Part model, mm, in its own coordinate system. A direction names the side the tool comes from. Round coordinates to 2 decimals unless told otherwise and drop trailing zeros. Write each loop counter-clockwise with the first axis right and the second up, starting at its lowest first coordinate (ties: lowest second). Pieces come first, ordered by that corner, then holes. Notation, with made-up numbers: (37, 63.25) -> (96, 63.25) arc R20 cw to (96, 96.25) -> close; hole circle Ø1 at (-32.5, 28). An arc over 180 degrees is marked (long way). Return JSON: item names as keys, results as strings. Group by question number.
```python
from build123d import *

# Parameters (mm, degrees)
SKETCH016_R      = 2.005
EXTRUDE074_DEPTH = 20
EXTRUDE073_DEPTH = 20
EXTRUDE072_DEPTH = 20
EXTRUDE071_DEPTH = 20
EXTRUDE070_DEPTH = 20
EXTRUDE069_DEPTH = 20
EXTRUDE068_DEPTH = 20
SKETCH015_R      = 2.5
EXTRUDE067_DEPTH = 8
SKETCH060_W      = 70
SKETCH060_H      = 6.56
EXTRUDE066_DEPTH = 70


with BuildPart() as tornillo015:
    # Sketch016 (on Face16 of Fusion001) → Extrude074 (new body)
    with BuildSketch(Plane.XY.offset(45.913223)):
        with Locations((-84.962639, 67.504814)):
            Circle(SKETCH016_R)
    extrude(amount=EXTRUDE074_DEPTH)


with BuildPart() as tornillo015_1:
    # Extrude074 placement: moved
    add(tornillo015.part.moved(Location((46.5, -21.8, -20.5))))


with BuildPart() as tornillo014:
    # Sketch016 (on Face16 of Fusion001) → Extrude073 (new body)
    with BuildSketch(Plane.XY.offset(45.913223)):
        with Locations((-84.962639, 67.504814)):
            Circle(SKETCH016_R)
    extrude(amount=EXTRUDE073_DEPTH)


with BuildPart() as tornillo014_1:
    # Extrude073 placement: moved
    add(tornillo014.part.moved(Location((23.6, -21.8, -20.6))))


with BuildPart() as tornillo013:
    # Sketch016 (on Face16 of Fusion001) → Extrude072 (new body)
    with BuildSketch(Plane.XY.offset(45.913223)):
        with Locations((-84.962639, 67.504814)):
            Circle(SKETCH016_R)
    extrude(amount=EXTRUDE072_DEPTH)


with BuildPart() as tornillo013_1:
    # Extrude072 placement: moved
    add(tornillo013.part.moved(Location((0, -21.8, -20.8))))


with BuildPart() as tornillo012:
    # Sketch016 (on Face16 of Fusion001) → Extrude071 (new body)
    with BuildSketch(Plane.XY.offset(45.913223)):
        with Locations((-84.962639, 67.504814)):
            Circle(SKETCH016_R)
    extrude(amount=EXTRUDE071_DEPTH)


with BuildPart() as tornillo012_1:
    # Extrude071 placement: moved
    add(tornillo012.part.moved(Location((0, -45, -17))))


with BuildPart() as tornillo011:
    # Sketch016 (on Face16 of Fusion001) → Extrude070 (new body)
    with BuildSketch(Plane.XY.offset(45.913223)):
        with Locations((-84.962639, 67.504814)):
            Circle(SKETCH016_R)
    extrude(amount=EXTRUDE070_DEPTH)


with BuildPart() as tornillo011_1:
    # Extrude070 placement: moved
    add(tornillo011.part.moved(Location((50, -45, -15))))


with BuildPart() as tornillo010:
    # Sketch016 (on Face16 of Fusion001) → Extrude069 (new body)
    with BuildSketch(Plane.XY.offset(45.913223)):
        with Locations((-84.962639, 67.504814)):
            Circle(SKETCH016_R)
    extrude(amount=EXTRUDE069_DEPTH)


with BuildPart() as tornillo010_1:
    # Extrude069 placement: moved
    add(tornillo010.part.moved(Location((0, 0, -15))))


with BuildPart() as tornillo009:
    # Sketch016 (on Face16 of Fusion001) → Extrude068 (new body)
    with BuildSketch(Plane.XY.offset(45.913223)):
        with Locations((-84.962639, 67.504814)):
            Circle(SKETCH016_R)
    extrude(amount=EXTRUDE068_DEPTH)


with BuildPart() as tornillo009_1:
    # Extrude068 placement: moved
    add(tornillo009.part.moved(Location((50.1, 0, -18))))


with BuildPart() as tornillos013:
    # Sketch015 (on Face16 of Fusion) → Extrude067 (new body)
    with BuildSketch(Plane.XY.offset(41.913223)):
        with Locations((-84.986267, 67.433998)):
            Circle(SKETCH015_R)
        with Locations((-85.013062, 22.499535)):
            Circle(SKETCH015_R)
        with Locations((-35.024185, 22.542374)):
            Circle(SKETCH015_R)
        with Locations((-34.910458, 67.59893)):
            Circle(SKETCH015_R)
    extrude(amount=EXTRUDE067_DEPTH)


with BuildPart() as tornillos013_1:
    # Extrude067 placement: moved
    add(tornillos013.part.moved(Location((0, 0, -4))))


with BuildPart() as obj1:
    # Sketch060 → Extrude066 (new body)
    with BuildSketch(Plane.YZ):
        with Locations((4.567114, 74.199239)):
            Rectangle(SKETCH060_W, SKETCH060_H)
    extrude(amount=EXTRUDE066_DEPTH)


with BuildPart() as obj1_1:
    # Extrude066 placement: moved
    add(obj1.part.moved(Location((-94.7, 41.5, -35.5))))

    # Fusion018: union Tornillos013
    add(tornillos013_1.part)

    # Cut036: cut Tornillo009
    add(tornillo009_1.part, mode=Mode.SUBTRACT)

    # Cut037: cut Tornillo010
    add(tornillo010_1.part, mode=Mode.SUBTRACT)

    # Cut038: cut Tornillo011
    add(tornillo011_1.part, mode=Mode.SUBTRACT)

    # Cut039: cut Tornillo012
    add(tornillo012_1.part, mode=Mode.SUBTRACT)

    # Cut040: cut Tornillo013
    add(tornillo013_1.part, mode=Mode.SUBTRACT)

    # Cut041: cut Tornillo014
    add(tornillo014_1.part, mode=Mode.SUBTRACT)

    # Cut042: cut Tornillo015
    add(tornillo015_1.part, mode=Mode.SUBTRACT)


solid = obj1_1.part
```
Item 1: Cut at D-D (x = -65.5). Write the cut outline in (y, z).
Item 2: Cut at C-C (z = 37.75). Write the cut outline in (x, y) (3 decimals), then the cut area to 3 significant figures.
Item 3: Wall check: L1, parallel to Y at x = -85, z = 37; L2, parallel to Y at x = -35, z = 38.25; L3, parallel to X at y = 69, z = 40.5. Give the ranges that are in metal, low to high.
Item 4: Flat gauge pin, fed straight in: P1, Ø6, axis at x = -77.5, y = 70, coming from the +Z side. Where does the tip first touch, or does it go through?
Item 5: Cut at B-B (x = -34). Write the cut outline in (y, z), then the cut area to 3 significant figures.
Item 6: Cut at A-A (z = 44). Write the cut outline in (x, y) (3 decimals).
Item 7: Two-plate mould, pull along Y, no slides. Class faces 1 (the face through (-60, 11.067, 39)), 2 (the face through (-94.7, 46, 39)), 3 (the face through (-84.037, 43.926, 38.653)): released by +Y, released by -Y, zero draft, split by the parting line, or undercut.
Item 8: Which spindle directions (+Z, -Z, +X, -X, +Y, -Y) get a long thin tool onto all of the face, cutting with end or side? Do faces 4 (the face through (-60, 38, 41.979)), 5 (the face through (-33.11, 21.74, 40.59)). Say none if no direction does.
Checks:
{
 "1": {"outline": "(11.07, 35.42) -> (81.07, 35.42) -> (81.07, 41.98) -> (11.07, 41.98) -> close"},
 "2": {"outline": "(-94.7, 11.067) -> (-24.7, 11.067) -> (-24.7, 81.067) -> (-94.7, 81.067) -> close; hole circle Ø4.01 at (-84.963, 22.505); hole circle Ø4.01 at (-84.963, 45.705); hole circle Ø4.01 at (-84.963, 67.505); hole circle Ø4.01 at (-61.363, 45.705); hole circle Ø4.01 at (-38.463, 45.705); hole circle Ø4.01 at (-34.963, 22.505); hole circle Ø4.01 at (-34.863, 67.505)", "area": "4,810 mm2"},
 "3": {"L1": "y = 11.07 to 20.5, 24.51 to 43.7, 47.71 to 65.5, 69.51 to 81.07", "L2": "y = 11.07 to 20.5, 24.51 to 65.5, 69.51 to 81.07", "L3": "x = -94.7 to -86.3, -83.63 to -36.2, -33.53 to -24.7"},
 "4": {"P1": "stops at z = 41.98"},
 "5": {"outline": "(11.07, 35.42) -> (20.75, 35.42) -> (20.75, 45.91) -> (20.26, 45.91) -> (20.26, 41.98) -> (11.07, 41.98) -> close; (24.26, 35.42) -> (65.69, 35.42) -> (65.69, 45.91) -> (65.27, 45.91) -> (65.27, 41.98) -> (24.82, 41.98) -> (24.82, 45.91) -> (24.26, 45.91) -> close; (69.31, 35.42) -> (81.07, 35.42) -> (81.07, 41.98) -> (69.93, 41.98) -> (69.93, 45.91) -> (69.31, 45.91) -> close", "area": "421 mm2"},
 "6": {"outline": "circle Ø5 at (-85.013, 22.5); circle Ø5 at (-84.986, 67.434); circle Ø5 at (-35.024, 22.542); circle Ø5 at (-34.91, 67.599); hole circle Ø4.01 at (-84.963, 22.505); hole circle Ø4.01 at (-84.963, 67.505); hole circle Ø4.01 at (-34.963, 22.505); hole circle Ø4.01 at (-34.863, 67.505)"},
 "7": {"face 1": "released by -Y", "face 2": "zero draft", "face 3": "undercut"},
 "8": {"face 4": "+Z", "face 5": "+Z, -Z"}
}
